The drawing under review shows one solid part. Ordinate dimensions are in mm from its lowest x, y, z. A direction names the side the tool comes from. Give positions to 0.01 mm unless a question says otherwise; leave off trailing zeros. Loops run counter-clockwise (first coordinate to the right, second up) from the corner with the lowest first, then second, coordinate; pieces in that order, holes last. Notation, with made-up numbers: M 89,7.5 L 98,7.5 A20 cw 98,39.5 Z; hole C 32.5,43 d10. An arc over 180 degrees is marked long. Write item = value, one per line. Start each with the question number.
1. For the marked faces 4 and 5, list the 3-axis set-ups (+Z, -Z, +X, -X, +Y, -Y) from which the entire face can be reached by the end or side of a thin tool; tool diameter is ignored.
2. We need section A-A on x = 13. Give the boundary of the cut face in (y, z), then the cut area to 3 significant figures.
3. We need section D-D on y = 10. Give the boundary of the cut face in (x, z).
4. Wall thickness on line 1 along Z through (x, y) = (13, 39.75) (3 decimals); line 2 along Y through (x, z) = (13, 9.75); line 3 along Z through (x, y) = (8.75, 39): over which ranges is each line inside the solid? List them lowest first. Write a range as from..to.
5. We need section B-B on y = 3.5. Give the boundary of the cut face in (x, z), then the cut area to 3 significant figures.
6. For pin 1 (2.5 mm diameter, centred on y = 3, z = 13.5, fed in from -X); pin 2 (6 mm diameter, centred on x = 19, y = 32, fed in from +Z); pin 3 (2.5 mm diameter, centred on x = 13, y = 3.5, fed in from +Z) (3 decimals); pin 4 (12.5 mm diameter, centred on x = 9.5, z = 18, fed in from +Y), all flat-tipped, find the tip position at first contact; note any pin that passes through.
7. We need section C-C on y = 20.5. Give the boundary of the cut face in (x, z), then the cut area to 3 significant figures.
8. Draft analysis for pull direction X (two halves, no side actions). For the marked faces 1, 2 and 3, state which applies: pulls with the +X half, pulls with the -X half, needs draft (parallel to the pull), parting line crosses it, or undercut.
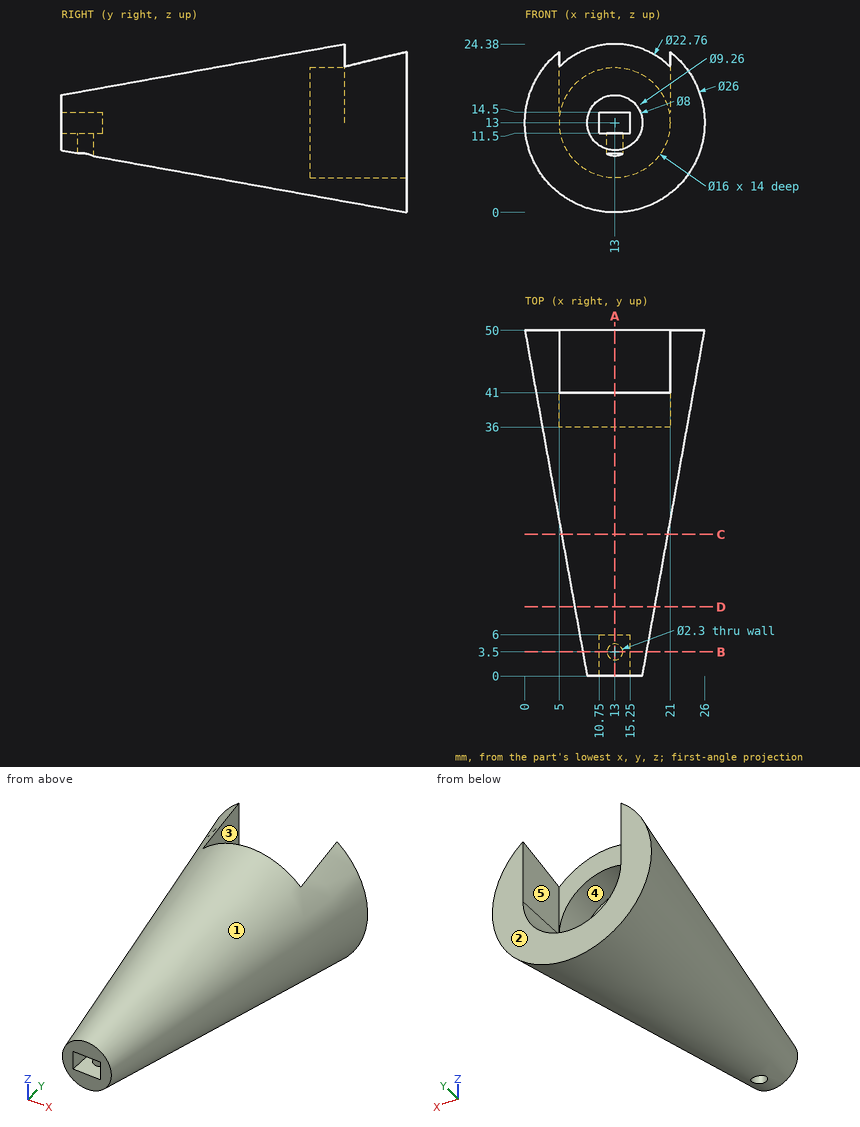
Final values:
q1.face_4 = +Y
q1.face_5 = +Z, +Y
q2.outline = M 0,9 L 2.35,8.58 L 2.35,11.5 L 0,11.5 Z; M 0,14.5 L 6,14.5 L 6,11.5 L 4.65,11.5 L 4.65,8.16 L 50,0 L 50,5 L 36,5 L 36,21 L 41,21 L 41,24.38 L 0,17 Z
q2.area = 563 mm²
q3.outline = C 13,13 d11.6
q4.line_1 = 1.845..5, 21..24.155
q4.line_2 = 0..2.35, 4.65..36
q4.line_3 = 2.83..6.22, 19.78..23.17
q5.outline = M 10.75,11.5 L 10.75,14.5 L 15.25,14.5 L 15.25,11.5 L 14.15,11.5 L 14.15,8.52 A4.63 ccw long 11.85,8.52 L 11.85,11.5 Z
q5.area = 46.8 mm²
q6.pin_1 = 8.25
q6.pin_2 = 22.44
q6.pin_3 = 17.855
q6.pin_4 = 50
q7.outline = C 13,13 d15.38
q7.area = 186 mm²
q8.face_1 = parting line crosses it
q8.face_2 = needs draft
q8.face_3 = undercut
